```python
from build123d import *

# Parameters (mm, degrees)
SKETCH_1_W      = 36
SKETCH_1_H      = 36
SKETCH_1_W_2    = 21.620111732
SKETCH_1_H_2    = 21.620111732
EXTRUDE_1_DEPTH = 10
SKETCH_1_3_W    = 21.620111732
SKETCH_1_3_H    = 21.620111732
EXTRUDE_2_DEPTH = 3
SKETCH_2_R      = 7.5
EXTRUDE_3_DEPTH = 8


with BuildPart() as part:
    # Sketch 1 → Extrude 1 (new body)
    # profile 1 of 2: a face of its own
    with BuildSketch(Plane.XY):
        Rectangle(SKETCH_1_W, SKETCH_1_H)
        Rectangle(SKETCH_1_W_2, SKETCH_1_H_2, mode=Mode.SUBTRACT)
    # profile 2 of 2: a face of its own
    with BuildSketch(Plane.XY):
        Rectangle(SKETCH_1_W_2, SKETCH_1_H_2)
    extrude(amount=EXTRUDE_1_DEPTH)

    # Sketch 1_3 → Extrude 2 (add)
    with BuildSketch(Plane.XY):
        Rectangle(SKETCH_1_3_W, SKETCH_1_3_H)
    extrude(amount=-EXTRUDE_2_DEPTH)

    # Sketch 2 → Extrude 3 (add)
    with BuildSketch(Plane(origin=(0, 0, -3), x_dir=(-1, 0, 0), z_dir=(0, 0, -1))):
        Circle(SKETCH_2_R)
    extrude(amount=EXTRUDE_3_DEPTH)


solid = part.part
```
Source: CAD feature listing. Evaluate the final solid. Frame: model axes, mm. A direction names the side the tool comes from. Give positions to 0.01 mm unless a question says otherwise; leave off trailing zeros. Order: outer loops, then holes, each group sorted by start corner. A loop starts at its lowest first (then second) coordinate and runs counter-clockwise, first axis right, second up.
(1) Contact query for flat-ended pins moving along their axis: P1, Ø2.5, axis at x = -1, z = -1.5, coming from the +Y side; P2, Ø6, axis at x = -4, z = -7, coming from the -Y side; P3, Ø12, axis at x = -13.5, y = -8, coming from the -Z side; P4, Ø3, axis at y = 9.5, z = -5, coming from the -X side. Output: stop coordinate, or through.
(2) Access query for faces 1 (the face through (0, 10.81, -1)), 2 (the face through (-10.81, 0, -1)), 3 (the face through (0, -10.81, -1)), 4 (the face through (-2.6, 7.4, -3)). Directions: +Z, -Z, +X, -X, +Y, -Y. A direction counts if a zero-diameter tool reaches every point of the face in a straight line with its end or side. Return the directions, or none.
(3) Section query D-D (y = -9). Return the cut outline in (x, z), plus the area to 3 significant figures.
(4) Section query C-C (z = -6.75). Return the cut outline in (x, y), plus the area to 3 significant figures.
(5) Section query A-A (y = 0). Return the cut outline in (x, z), plus the area to 3 significant figures.
(6) Material intervals for line 1 along Z through (x, y) = (10, -9); line 2 along Z through (x, y) = (-11, -9); line 3 along Y through (x, z) = (9, -0.25), sorted ascending.
(7) Section query B-B (x = 0.5). Return the cut outline in (y, z).
Outcome:
1. P1: stops at y = 10.81
1. P2: stops at y = -7.43
1. P3: stops at z = -3
1. P4: passes through
2. face 1: -Z, +X, -X, +Y
2. face 2: -Z, -X, +Y, -Y
2. face 3: -Z, +X, -X, -Y
2. face 4: -Z
3. outline: (-18, 0) - (-10.81, 0) - (-10.81, -3) - (10.81, -3) - (10.81, 0) - (18, 0) - (18, 10) - (-18, 10) - close
3. area: 425 mm2
4. outline: circle Ø15 at (0, 0)
4. area: 177 mm2
5. outline: (-18, 0) - (-10.81, 0) - (-10.81, -3) - (-7.5, -3) - (-7.5, -11) - (7.5, -11) - (7.5, -3) - (10.81, -3) - (10.81, 0) - (18, 0) - (18, 10) - (-18, 10) - close
5. area: 545 mm2
6. line 1: z = -3 to 10
6. line 2: z = 0 to 10
6. line 3: y = -10.81 to 10.81
7. outline: (-18, 0) - (-10.81, 0) - (-10.81, -3) - (-7.48, -3) - (-7.48, -11) - (7.48, -11) - (7.48, -3) - (10.81, -3) - (10.81, 0) - (18, 0) - (18, 10) - (-18, 10) - close
